Can you work these out from the drawing? Everything is in mm from the part's minimum corner. A direction names the side the tool comes from. Give positions to 0.01 mm unless a question says otherwise; leave off trailing zeros. Loops run counter-clockwise (first coordinate to the right, second up) from the corner with the lowest first, then second, coordinate; pieces in that order, holes last. Notation, with made-up numbers: (-20, 79.25) - (-10, 79.25) arc R16 cw to (-10, 88.25) - close; hole circle Ø11 at (14, 39). An arc over 180 degrees is marked (long way). Answer in a Markdown table with one row per item.
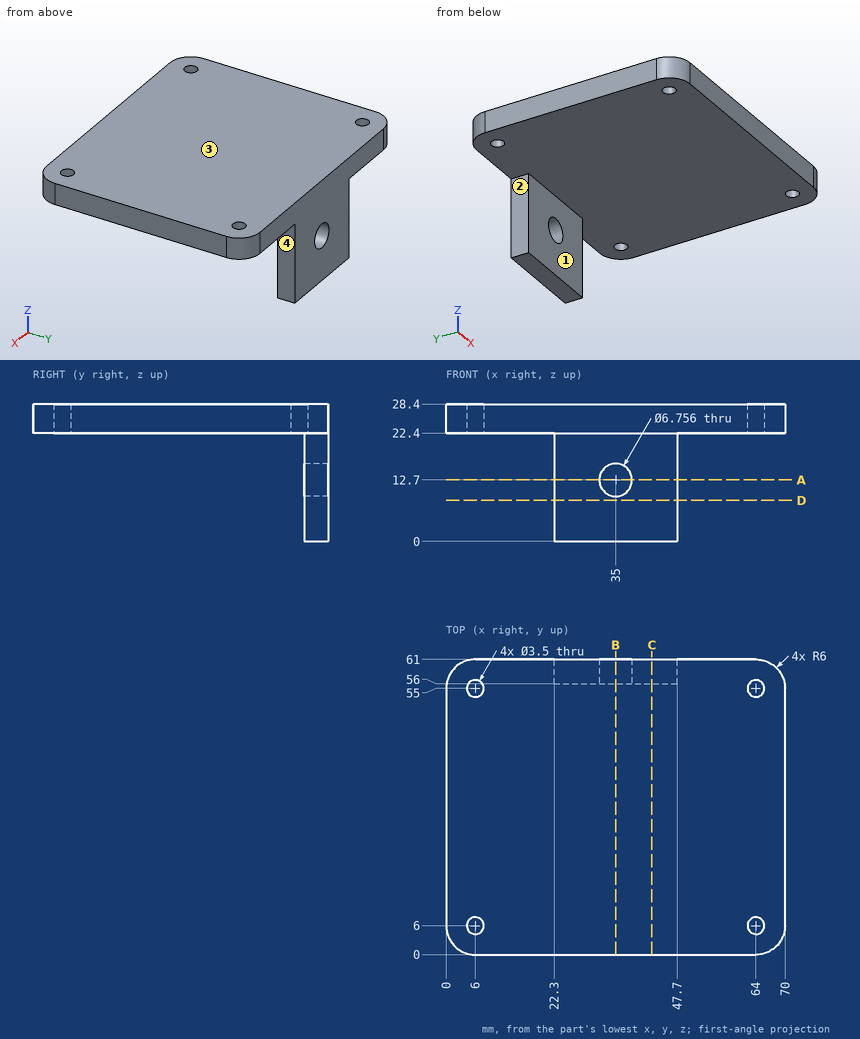
Q1. Imagine slicing it at A-A, the plane z = 12.7. Write out the boundary of the cut face in (x, y).
Checked values:
| item | result |
|---|---|
| outline | (22.3, 56) - (31.62, 56) - (31.62, 61) - (22.3, 61) - close; (38.38, 56) - (47.7, 56) - (47.7, 61) - (38.38, 61) - close |
Q2. On a 3-axis mill with a long thin cutter (end or side, diameter ignored), from which of +Z, -Z, +X, -X, +Y, -Y can I reach the whole of each face in a straight line? I mean the marked faces 1, 2, 3 and 4. Say none if no direction works.
Checked values:
| item | result |
|---|---|
| face 1 | -Z, +X, -X, -Y |
| face 2 | -Z, -X, +Y, -Y |
| face 3 | +Z, +X, -X, +Y, -Y |
| face 4 | -Z, +X, +Y, -Y |
Q3. Imagine slicing it at D-D, the plane z = 8.5. Write out the boundary of the cut face in (x, y).
Checked values:
| item | result |
|---|---|
| outline | (22.3, 56) - (47.7, 56) - (47.7, 61) - (22.3, 61) - close |
Q4. If I drill on line 1 (Y direction, x = 64, z = 26.75); line 2 (Z direction, x = 38, y = 5); line 3 (Z direction, x = 35, y = 59), over which ranges is the centre line in solid material (lowest first)? Write a range as [from, to].
Checked values:
| item | result |
|---|---|
| line 1 | y = [0, 4.25], [7.75, 53.25], [56.75, 61] |
| line 2 | z = [22.4, 28.4] |
| line 3 | z = [0, 9.32], [16.08, 28.4] |
Q5. For pin 1 (4 mm diameter, centred on x = 6, y = 6, fed in from -Z); pin 2 (8 mm diameter, centred on y = 23.5, z = 19.5, fed in from +X); pin 3 (4 mm diameter, centred on y = 58, z = 5.5, fed in from -X); pin 4 (6 mm diameter, centred on y = 53.5, z = 16.5, fed in from +X), each with a flat end and sliding along its axis, tell me the tip position at first contact or that it passes through.
Checked values:
| item | result |
|---|---|
| pin 1 | stops at z = 22.4 |
| pin 2 | stops at x = 70 |
| pin 3 | stops at x = 22.3 |
| pin 4 | stops at x = 47.7 |
Q6. Imagine slicing it at B-B, the plane x = 35. Write out the boundary of the cut face in (y, z).
Checked values:
| item | result |
|---|---|
| outline | (0, 22.4) - (56, 22.4) - (56, 16.08) - (61, 16.08) - (61, 28.4) - (0, 28.4) - close; (56, 0) - (61, 0) - (61, 9.32) - (56, 9.32) - close |
Q7. Imagine slicing it at C-C, the plane x = 42.5. Write out the boundary of the cut face in (y, z).
Checked values:
| item | result |
|---|---|
| outline | (0, 22.4) - (56, 22.4) - (56, 0) - (61, 0) - (61, 28.4) - (0, 28.4) - close |
